from build123d import *

# Parameters (mm, degrees)
SKETCH_R           = 13.75
SKETCH_R_2         = 12.325
PAD_DEPTH          = 15.5
SKETCH001_R        = 17.5
PAD001_DEPTH       = 1.5
CHAMFER_SIZE2      = 2
CHAMFER_SIZE       = 0.7
SKETCH002_R        = 0.5
POCKET_DEPTH       = 122.171913
POCKET_DEPTH_BACK  = 122.171913
POLARPATTERN_COUNT = 2
POLARPATTERN_ANGLE = 90


with BuildPart() as part:
    # Sketch → Pad (new body)
    with BuildSketch(Plane.XY):
        Circle(SKETCH_R)
        Circle(SKETCH_R_2, mode=Mode.SUBTRACT)
    extrude(amount=PAD_DEPTH)

    # Sketch001 → Pad001 (join)
    with BuildSketch(Plane.XY):
        Circle(SKETCH001_R)
    extrude(amount=-PAD001_DEPTH)

    # Chamfer
    chamfer_edges = [part.edges().sort_by_distance(p)[0] for p in [
        (-12.325, 0, 15.5),
    ]]
    chamfer_side = part.faces().sort_by_distance((-13.361091, 0, 15.5))[0]
    chamfer(chamfer_edges, length=CHAMFER_SIZE, length2=CHAMFER_SIZE2, reference=chamfer_side)

    # Sketch002 → Pocket (cut, two sides)
    with BuildSketch(Plane.YZ) as pocket_sk:
        Circle(SKETCH002_R)
    pocket = extrude(amount=-POCKET_DEPTH, mode=Mode.SUBTRACT) + extrude(pocket_sk.sketch, amount=POCKET_DEPTH_BACK, mode=Mode.SUBTRACT)

    # PolarPattern: Pocket ×2 about axis
    polarpattern_axis = Axis((0, 0, 0), (0, 0, 1))
    for i in range(1, POLARPATTERN_COUNT):
        add(pocket.rotate(polarpattern_axis, i * POLARPATTERN_ANGLE / (POLARPATTERN_COUNT - 1)), mode=Mode.SUBTRACT)


solid = part.part
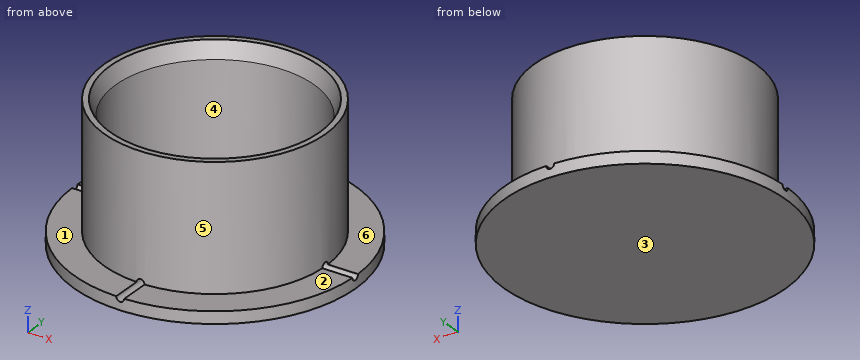
Read the model definition and answer for the solid it produces. Units are mm, in the model's axes. Face numbers are marked on the shaded views. A direction names the side the tool comes from. Coordinates: 2 decimals unless noted, no trailing zeros. Loops run counter-clockwise (first coordinate to the right, second up) from the corner with the lowest first, then second, coordinate; pieces in that order, holes last.
Q1. Each of these flat-tipped pins is pushed along its axis until it touches: pin 1 Ø5 at (x, y) = (-4, -7) entering from +Z; pin 2 Ø2 at (x, z) = (-12.5, 10.5) entering from -Y; pin 3 Ø1 at (x, z) = (10.5, 5) entering from +Y. Where does it stop, or does it pass through?
Q2. Consider probe 1 along X at (y, z) = (0, 6.75) (3 decimals); probe 2 along Y at (x, z) = (4, 1.5). Determine where each line is inside the solid, lowest interval first.
Q3. The mould has two halves that part along X. Classify the marked faces 4, 5 and 6: +X half, -X half, draft (parallel to the pull), parting line (faces both ways), or undercut.
Q4. The part is cut by section A-A on z = 8.25. Write down the section's boundary in (x, y) (3 decimals).
Q5. Which of the six approach directions +Z, -Z, +X, -X, +Y, -Y give full straight-line access (tool end or side, diameter ignored) to the marked faces 1, 2 and 3?
Results below:
1. pin 1: stops at z = 0
1. pin 2: stops at y = -7.54
1. pin 3: stops at y = 9.44
2. probe 1: x = -13.75 to -12.325, 12.325 to 13.75
2. probe 2: y = -13.16 to -11.66, 11.66 to 13.16
3. face 4: undercut
3. face 5: parting line
3. face 6: draft
4. outline: circle Ø27.5 at (0, 0); hole circle Ø24.65 at (0, 0)
5. face 1: +Z, -X, -Y
5. face 2: +Z, +X, -Y
5. face 3: -Z, +X, -X, +Y, -Y
